```python
from build123d import *

# Parameters (mm, degrees)
PACKAGING_START                     = -2.65
SKETCH2_W                           = 8
SKETCH2_H                           = 11.4
PACKAGING_FLAT_AT_Z_MINUS2P65_DEPTH = 20


with BuildPart() as part:
    # Sketch1 → Revolve1 (revolve)
    with BuildSketch(Plane.XY, mode=Mode.PRIVATE) as revolve1_sk:
        Polygon((2.665, -18), (2.665, -5), (0.55, -5), (0.55, 11.4), (3.175, 11.4), (3.175, 0), (4.619, 0), (4.619, -3), (3.24, -3), (3.24, -18), align=None)
    revolve(revolve1_sk.sketch.rotate(Axis((0, -200, 0), (0, 1, 0)), 90), axis=Axis((0, -200, 0), (0, 1, 0)))

    # Sketch2 → Packaging flat at Z minus2p65 (cut)
    with BuildSketch(Plane.XY.offset(PACKAGING_START)):
        with Locations((0, 5.7)):
            Rectangle(SKETCH2_W, SKETCH2_H)
    extrude(amount=-PACKAGING_FLAT_AT_Z_MINUS2P65_DEPTH, mode=Mode.SUBTRACT)


solid = part.part
```
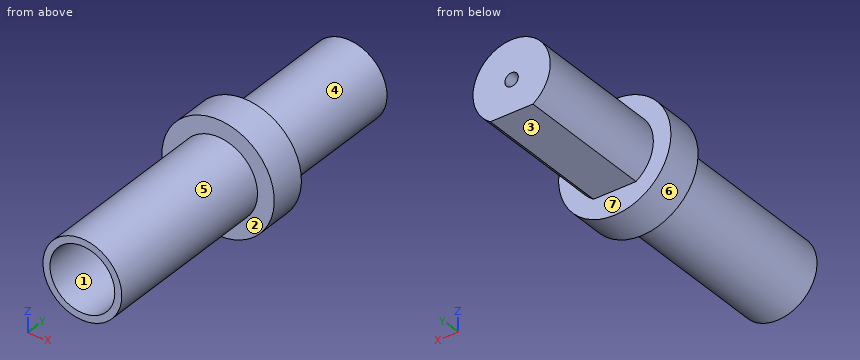
The listing builds one solid part. Answer for the finished solid, in the listing's coordinates (mm). Face numbers are marked on the shaded views. A direction names the side the tool comes from. Coordinates: 2 decimals unless noted, no trailing zeros. Loops run counter-clockwise (first coordinate to the right, second up) from the corner with the lowest first, then second, coordinate; pieces in that order, holes last. Notation, with made-up numbers: (-6, -35) - (18, -35) arc R11 cw to (18, -26) - close; hole circle Ø6 at (25, 69). An arc over 180 degrees is marked (long way). Write item = value, one per line.
1) Section D-D (z = 2) is taken. Determine the outline of the cut face in (x, y).
Responses:
outline = (-4.16, -3) - (-2.55, -3) - (-2.55, -18) - (-1.76, -18) - (-1.76, -5) - (1.76, -5) - (1.76, -18) - (2.55, -18) - (2.55, -3) - (4.16, -3) - (4.16, 0) - (2.47, 0) - (2.47, 11.4) - (-2.47, 11.4) - (-2.47, 0) - (-4.16, 0) - close
2) Each of these flat-tipped pins is pushed along its axis until it touches: P1, Ø1.6, axis at x = -0.5, z = -0.5, coming from the -Y side; P2, Ø2, axis at y = -6, z = -1, coming from the +X side; P3, Ø4, axis at x = 1, y = 6, coming from the -Z side. Where does it stop, or does it pass through?
Responses:
P1 = -5
P2 = 3.24
P3 = -2.65
3) Section C-C (y = -6.5) is taken. Determine the outline of the cut face in (x, z) (3 decimals).
Responses:
outline = circle Ø6.48 at (0, 0); hole circle Ø5.33 at (0, 0)
4) Determine the mould class of the marked faces 1, 2, 3 and 4 for opening direction Z: pulls with the +Z half, pulls with the -Z half, needs draft (parallel to the pull), parting line crosses it, or undercut.
Responses:
face_1 = undercut
face_2 = needs draft
face_3 = pulls with the -Z half
face_4 = parting line crosses it
5) Section B-B (x = 0) is taken. Determine the outline of the cut face in (y, z) (3 decimals), plus the area to 3 significant figures.
Responses:
outline = (-18, -3.24) - (-3, -3.24) - (-3, -4.619) - (0, -4.619) - (0, -2.65) - (11.4, -2.65) - (11.4, -0.55) - (-5, -0.55) - (-5, -2.665) - (-18, -2.665) - close; (-18, 2.665) - (-5, 2.665) - (-5, 0.55) - (11.4, 0.55) - (11.4, 3.175) - (0, 3.175) - (0, 4.619) - (-3, 4.619) - (-3, 3.24) - (-18, 3.24) - close
area = 104 mm^2
6) Find the intervals of material crossed by line 1 along X through (y, z) = (-8.5, 0) (3 decimals); line 2 along X through (y, z) = (1, 0) (3 decimals); line 3 along Y through (x, z) = (-0.25, -3), in increasing order.
Responses:
line_1 = -3.24 to -2.665, 2.665 to 3.24
line_2 = -3.175 to -0.55, 0.55 to 3.175
line_3 = -18 to 0
7) Which of the six approach directions +Z, -Z, +X, -X, +Y, -Y give full straight-line access (tool end or side, diameter ignored) to the marked faces 5, 6 and 7?
Responses:
face_5 = -Y
face_6 = +Y, -Y
face_7 = +Y
8) Section A-A (z = 0) is taken. Determine the outline of the cut face in (x, y) (3 decimals), plus the area to 3 significant figures.
Responses:
outline = (-4.619, -3) - (-3.24, -3) - (-3.24, -18) - (-2.665, -18) - (-2.665, -5) - (-0.55, -5) - (-0.55, 11.4) - (-3.175, 11.4) - (-3.175, 0) - (-4.619, 0) - close; (0.55, -5) - (2.665, -5) - (2.665, -18) - (3.24, -18) - (3.24, -3) - (4.619, -3) - (4.619, 0) - (3.175, 0) - (3.175, 11.4) - (0.55, 11.4) - close
area = 110 mm^2
